Source: CAD feature listing. Evaluate the final solid. Frame: model axes, mm. Give positions to 0.01 mm unless a question says otherwise; leave off trailing zeros. Loops run counter-clockwise (first coordinate to the right, second up) from the corner with the lowest first, then second, coordinate; pieces in that order, holes last. Notation, with made-up numbers: (59, -8.5) -> (106, -8.5) arc R18 cw to (106, 9.5) -> close; hole circle Ø1 at (59.25, 28.25). An arc over 180 degrees is marked (long way). Return JSON: item names as keys, results as strings. Group by question number.
```python
from build123d import *

# Parameters (mm, degrees)
SKETCH1_R           = 90
BOSS_EXTRUDE1_DEPTH = 100


with BuildPart() as part:
    # Sketch1 → Boss-Extrude1 (new body)
    with BuildSketch(Plane(origin=(0, 0, 0), x_dir=(1, 0, 0), z_dir=(0, 1, 0))):
        with BuildLine():
            ThreePointArc((233.238075794, 90), (-250, 0), (233.238075794, -90))
            Line((233.238075794, -90), (782.991924206, -90))
            ThreePointArc((782.991924206, -90), (1016.23, -250), (1249.468075794, -90))
            Line((1249.468075794, -90), (1799.221924206, -90))
            ThreePointArc((1799.221924206, -90), (2282.46, 0), (1799.221924206, 90))
            Line((1799.221924206, 90), (1249.468075794, 90))
            ThreePointArc((1249.468075794, 90), (1016.23, 250), (782.991924206, 90))
            Line((782.991924206, 90), (233.238075794, 90))
        make_face()
        with Locations(Location((1016.23, 0, 0), (0, 0, 270))):
            Circle(SKETCH1_R, mode=Mode.SUBTRACT)
        with Locations(Location((0, 0, 0), (0, 0, 270))):
            Circle(SKETCH1_R, mode=Mode.SUBTRACT)
        with Locations(Location((2032.46, 0, 0), (0, 0, 270))):
            Circle(SKETCH1_R, mode=Mode.SUBTRACT)
    extrude(amount=BOSS_EXTRUDE1_DEPTH)


solid = part.part
```
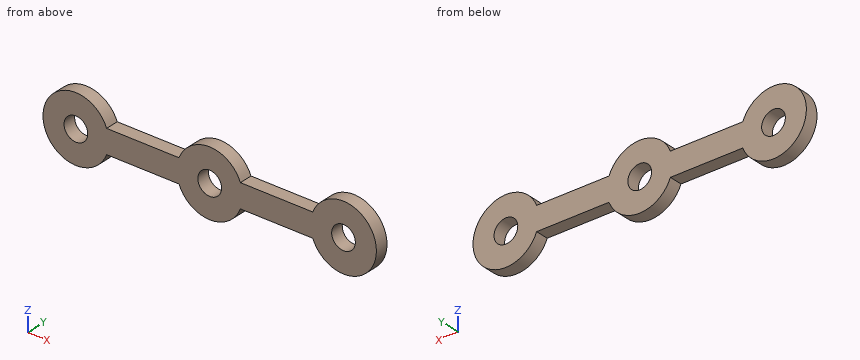
1) Cut plane A-A on x = 0. Return loops of the section in (y, z), then the cut area to 3 significant figures.
2) Material intervals for line 1 (X direction, y = 61, z = 0); line 2 (X direction, y = 64.5, z = -216); line 3 (X direction, y = 72, z = 53.5), sorted ascending.
3) Contact query for flat-ended pins moving along their axis: P1, Ø12, axis at y = 77, z = -102.5, coming from the -X side; P2, Ø1, axis at y = 55.5, z = 67.5, coming from the +X side; P3, Ø3, axis at y = 52, z = -48.5, coming from the -X side. Output: stop coordinate, or through.
4) Cut plane D-D on z = 193. Return loops of the section in (x, y).
5) Cut plane B-B on z = 0. Return loops of the section in (x, y), then the cut area to 3 significant figures.
6) Cut plane C-C on y = 34.5. Return loops of the section in (x, z), then the cut area to 3 significant figures.
Calculated:
{
 "1": {"outline": "(0, -250) -> (100, -250) -> (100, -90) -> (0, -90) -> close; (0, 90) -> (100, 90) -> (100, 250) -> (0, 250) -> close", "area": "32,000 mm2"},
 "2": {"line 1": "-250 to -90, 90 to 926.23, 1106.23 to 1942.46, 2122.46 to 2282.46", "line 2": "-125.87 to 125.87, 890.36 to 1142.1, 1906.59 to 2158.33", "line 3": "-244.21 to -72.37, 72.37 to 943.86, 1088.6 to 1960.09, 2104.83 to 2276.67"},
 "3": {"P1": "x = -230.62", "P2": "x = 2273.31", "P3": "x = -245.54"},
 "4": {"outline": "(-158.91, 0) -> (158.91, 0) -> (158.91, 100) -> (-158.91, 100) -> close; (857.32, 0) -> (1175.14, 0) -> (1175.14, 100) -> (857.32, 100) -> close; (1873.55, 0) -> (2191.37, 0) -> (2191.37, 100) -> (1873.55, 100) -> close"},
 "5": {"outline": "(-250, 0) -> (-90, 0) -> (-90, 100) -> (-250, 100) -> close; (90, 0) -> (926.23, 0) -> (926.23, 100) -> (90, 100) -> close; (1106.23, 0) -> (1942.46, 0) -> (1942.46, 100) -> (1106.23, 100) -> close; (2122.46, 0) -> (2282.46, 0) -> (2282.46, 100) -> (2122.46, 100) -> close", "area": "199,000 mm2"},
 "6": {"outline": "(233.24, -90) -> (782.99, -90) arc R250 ccw to (1249.47, -90) -> (1799.22, -90) arc R250 ccw (long way) to (1799.22, 90) -> (1249.47, 90) arc R250 ccw to (782.99, 90) -> (233.24, 90) arc R250 ccw (long way) to start; hole circle Ø180 at (0, 0); hole circle Ø180 at (1016.23, 0); hole circle Ø180 at (2032.46, 0)", "area": "703,000 mm2"}
}
